from build123d import *

# Parameters (mm, degrees)
SKETCH1_W                = 300
SKETCH1_H                = 230
BOSS_EXTRUDE1_DEPTH      = 50
CUT_EXTRUDE1_DEPTH       = 30
BOSS_EXTRUDE2_DEPTH      = 186
BOSS_EXTRUDE2_DEPTH_BACK = 431
SKETCH3_R                = 17.5


with BuildPart() as part:
    # Sketch1 → Boss-Extrude1 (new body)
    with BuildSketch(Plane(origin=(0, 0, 0), x_dir=(1, 0, 0), z_dir=(0, 1, 0))):
        Rectangle(SKETCH1_W, SKETCH1_H)
    extrude(amount=BOSS_EXTRUDE1_DEPTH)

    # Sketch2 → Cut-Extrude1 (cut)
    with BuildSketch(Plane(origin=(0, 50, 0), x_dir=(1, 0, 0), z_dir=(0, 1, 0))):
        with BuildLine():
            Line((116.702187757, 103.747196066), (-116.702187757, 103.747196066))
            ThreePointArc((-116.702187757, 103.747196066), (-130.844323381, 97.889331689), (-136.702187757, 83.747196066))
            Line((-136.702187757, 83.747196066), (-136.702187757, -83.747196066))
            ThreePointArc((-136.702187757, -83.747196066), (-130.844323381, -97.889331689), (-116.702187757, -103.747196066))
            Line((-116.702187757, -103.747196066), (116.702187757, -103.747196066))
            ThreePointArc((116.702187757, -103.747196066), (130.844323381, -97.889331689), (136.702187757, -83.747196066))
            Line((136.702187757, -83.747196066), (136.702187757, 83.747196066))
            ThreePointArc((136.702187757, 83.747196066), (130.844323381, 97.889331689), (116.702187757, 103.747196066))
        make_face()
    extrude(amount=-CUT_EXTRUDE1_DEPTH, mode=Mode.SUBTRACT)

    # Sketch3 → Boss-Extrude2 (add, two sides: drawn at the far end of the back side and taken through both)
    with BuildSketch(Plane(origin=(150, 0, 0), x_dir=(0, 0, -1), z_dir=(1, 0, 0)).offset(-BOSS_EXTRUDE2_DEPTH_BACK)):
        with Locations((115, 25)):
            Circle(SKETCH3_R)
        with Locations((-115, 25)):
            Circle(SKETCH3_R)
    extrude(amount=BOSS_EXTRUDE2_DEPTH + BOSS_EXTRUDE2_DEPTH_BACK)


solid = part.part
The model under review builds one solid part; all positions refer to its coordinate system, in mm. A direction names the side the tool comes from. Round coordinates to 2 decimals unless told otherwise and drop trailing zeros. Loops run counter-clockwise (first coordinate to the right, second up) from the corner with the lowest first, then second, coordinate; pieces in that order, holes last. Notation, with made-up numbers: (25, -28.5) - (43, -28.5) arc R20 cw to (43, -9.5) - close; hole circle Ø6 at (39, -27). An arc over 180 degrees is marked (long way). Use CSV: the item, a comma, the result in double quotes.
(1) For line 1 (X direction, y = 45.5, z = -33); line 2 (X direction, y = 18, z = 78); line 3 (Z direction, x = 61, y = 31.5), list the stretches that pass through material, from the lowest coordinate up.
Working result:
line 1,"x = -150 to -136.7, 136.7 to 150"
line 2,"x = -150 to 150"
line 3,"z = -131.25 to -98.75, 98.75 to 131.25"
(2) Take a section at A-A, the plane x = 107.5. Give the boundary of the cut face in (y, z).
Working result:
outline,"(0, -115) - (7.5, -115) arc R17.5 ccw to (42.5, -115) - (50, -115) - (50, -103.75) - (38.4, -103.75) arc R17.5 ccw to (20, -98.23) - (20, 98.23) arc R17.5 ccw to (38.4, 103.75) - (50, 103.75) - (50, 115) - (42.5, 115) arc R17.5 ccw to (7.5, 115) - (0, 115) - close"
(3) Clearance check with flat-ended pins moving along their axes: P1, Ø6, axis at x = -71, y = 15, coming from the -Z side; P2, Ø2, axis at x = 183.5, y = 24, coming from the +Z side; P3, Ø8, axis at x = -183, y = 17.5, coming from the -Z side; P4, Ø2, axis at x = -163.5, y = 12, coming from the +Z side. State where each tip first meets the part, or that it passes through.
Working result:
P1,"stops at z = -131.04"
P2,"stops at z = 132.5"
P3,"stops at z = -132.15"
P4,"stops at z = 127.74"
(4) Take a section at C-C, the plane x = -188. Give the boundary of the cut face in (y, z), plus the area to 3 significant figures.
Working result:
outline,"circle Ø35 at (25, -115); circle Ø35 at (25, 115)"
area,"1,920 mm^2"
(5) The part is to be moulded in two halves that separate along X. For faces 1 (the cylindrical face through (-1.8, 29.9, 98.2)), 2 (the flat face through (-150, 25, 2)), 3 (the flat face through (-1, 50, -111)), say which applies: pulls with the +X half, pulls with the -X half, needs draft (parallel to the pull), parting line crosses it, or undercut.
Working result:
face 1,"undercut"
face 2,"pulls with the -X half"
face 3,"needs draft"
(6) Take a section at B-B, the plane z = 64. Give the boundary of the cut face in (x, y), plus the area to 3 significant figures.
Working result:
outline,"(-150, 0) - (150, 0) - (150, 50) - (136.7, 50) - (136.7, 20) - (-136.7, 20) - (-136.7, 50) - (-150, 50) - close"
area,"6,800 mm^2"
(7) Machinability: for faces 4 (the flat face through (336, 25, 115)), 5 (the flat face through (136.702, 35, 1)), 6 (the cylindrical face through (23.181, 25.769, 132.483)), which of the approach directions +Z, -Z, +X, -X, +Y, -Y give a long, thin tool a straight path to every point of the face, cutting with its end or side? Answer none if there is none.
Working result:
face 4,"+Z, -Z, +X, +Y, -Y"
face 5,"+Y"
face 6,"none"
